from build123d import *

# Parameters (mm, degrees)
F0_W     = 20
F0_H     = 8.5
F1_DEPTH = 6


with BuildPart() as f1:
    # F0 (on Right) → F1 (new body)
    with BuildSketch(Plane.YZ):
        Polygon((0, 25), (0, 0), (0, -20), (300, -20), (300, 0), (300, 180), (300, 205), (240, 205), align=None)
        with Locations((30, 0)):
            Rectangle(F0_W, F0_H, mode=Mode.SUBTRACT)
        with Locations((90, 45)):
            Rectangle(F0_W, F0_H, mode=Mode.SUBTRACT)
        with Locations((150, 90)):
            Rectangle(F0_W, F0_H, mode=Mode.SUBTRACT)
        with Locations((210, 135)):
            Rectangle(F0_W, F0_H, mode=Mode.SUBTRACT)
        with Locations((270, 180)):
            Rectangle(F0_W, F0_H, mode=Mode.SUBTRACT)
    extrude(amount=F1_DEPTH)


solid = f1.part
Read the model definition and answer for the solid it produces. Units are mm, in the model's axes. A direction names the side the tool comes from. Coordinates: 2 decimals unless noted, no trailing zeros. Order: outer loops, then holes, each group sorted by start corner. A loop starts at its lowest first (then second) coordinate and runs counter-clockwise, first axis right, second up. Notation, with made-up numbers: M 68.25,47.5 L 90.25,47.5 A17 cw 90.25,71.5 Z; hole C -20,39.25 d3. An arc over 180 degrees is marked long. Put each result on its own line as item: value. Start each with the question number.
Item 1: Consider probe 1 along Z at (x, y) = (0.9, 84.5) (3 decimals); probe 2 along Z at (x, y) = (3.5, 204); probe 3 along Y at (x, z) = (3.9, 130). Determine where each line is inside the solid, lowest interval first. Write a range as [from, to].
Item 2: Section C-C, the plane z = 71.5 is taken. Determine the outline of the cut face in (x, y).
Item 3: For faces 4 (the face through (3, 20, 0)), 5 (the face through (0, 181, 69)), determine the directions among +Z, -Z, +X, -X, +Y, -Y from which every point of the face is accessible in a straight line to the end or side of a thin tool.
Item 4: The mould has two halves that part along Z. Classify faces 1 (the face through (3, 100, 45)), 2 (the face through (3, 0, 3)), 3 (the face through (3, 270, 205)): +Z half, -Z half, draft (parallel to the pull), parting line (faces both ways), or undercut.
Item 5: Section B-B, the plane x = 4.25 is taken. Determine the outline of the cut face in (y, z).
Item 6: Section D-D, the plane y = 135 is taken. Determine the outline of the cut face in (x, z).
Item 7: Given pin 1 Ø1.8 at (x, y) = (3, 213) entering from +Z (3 decimals); pin 2 Ø1.5 at (x, z) = (4, 118) entering from -Y; pin 3 Ø3 at (x, y) = (3, 209.5) entering from +Z, each flat-ended and moving along its own axis, determine where each tip first touches the part or whether it passes through.
Item 8: Section A-A, the plane y = 263.5 is taken. Determine the outline of the cut face in (x, z), plus the area to 3 significant figures.
Computed:
1. probe 1: z = [-20, 40.75], [49.25, 88.375]
1. probe 2: z = [-20, 130.75], [139.25, 178]
1. probe 3: y = [140, 300]
2. outline: M 0,62 L 6,62 L 6,300 L 0,300 Z
3. face 4: +X, -X
3. face 5: +Z, -Z, -X, +Y, -Y
4. face 1: undercut
4. face 2: draft
4. face 3: +Z half
5. outline: M 0,-20 L 300,-20 L 300,205 L 240,205 L 0,25 Z; hole M 20,-4.25 L 40,-4.25 L 40,4.25 L 20,4.25 Z; hole M 80,40.75 L 100,40.75 L 100,49.25 L 80,49.25 Z; hole M 140,85.75 L 160,85.75 L 160,94.25 L 140,94.25 Z; hole M 200,130.75 L 220,130.75 L 220,139.25 L 200,139.25 Z; hole M 260,175.75 L 280,175.75 L 280,184.25 L 260,184.25 Z
6. outline: M 0,-20 L 6,-20 L 6,126.25 L 0,126.25 Z
7. pin 1: stops at z = 185.425
7. pin 2: stops at y = 123
7. pin 3: stops at z = 183.25
8. outline: M 0,-20 L 6,-20 L 6,175.75 L 0,175.75 Z; M 0,184.25 L 6,184.25 L 6,205 L 0,205 Z
8. area: 1,300 mm2
